The model under review builds one solid part; all positions refer to its coordinate system, in mm. Face numbers are marked on the shaded views. A direction names the side the tool comes from. Round coordinates to 2 decimals unless told otherwise and drop trailing zeros. Write each loop counter-clockwise with the first axis right and the second up, starting at its lowest first coordinate (ties: lowest second). Pieces come first, ordered by that corner, then holes. Notation, with made-up numbers: (17.25, -39.5) -> (44.25, -39.5) arc R25 cw to (44.25, -3.5) -> close; hole circle Ø9 at (-16, 44.25). An arc over 180 degrees is marked (long way). Answer as a JSON object with one key per item and string values. Group by question number.
1) Mouldability with a two-part tool opening along X and no side actions: class the marked faces 6, 7, 8 and 9 as pulls with the +X half, pulls with the -X half, needs draft (parallel to the pull), parting line crosses it, or undercut.
2) We need section C-C, the plane z = 15. Count the separate pieces of the cut face and the enclosed holes in it, then the cut area to 3 significant figures.
3) Machinability: for the marked faces 1, 2, 3, 4 and 5, which of the approach directions +Z, -Z, +X, -X, +Y, -Y give a long, thin tool a straight path to every point of the face, cutting with its end or side? Answer none if there is none.
4) We need section D-D, the plane x = 23. Write out the cut boundary in (y, z), then the cut area to 3 significant figures.
5) We need section A-A, the plane x = 18. Write out the cut boundary in (y, z).
6) We need section B-B, the plane y = 11.25. Write out the cut boundary in (x, z).
7) Insertion check: pin 1 Ø4 at (x, y) = (14.5, 6.5) entering from +Z; pin 2 Ø6 at (x, z) = (23, 21) entering from -Y; pin 3 Ø5 at (x, y) = (18.5, 6.5) entering from +Z. Each pin has a flat end and moves straight along its axis. Give the tip position at first contact, or say it passes through.
8) To check wall thickness, follow probe 1 along Y at (x, z) = (18, 4.65); probe 2 along Y at (x, z) = (18, 1.6); probe 3 along X at (y, z) = (21.25, 18.5). State the ranges of each line that lie inside material, in increasing order. Write a range as [from, to].
from build123d import *

# Parameters (mm, degrees)
SKETCH1_W                                           = 36
SKETCH1_H                                           = 24
BOSS_EXTRUDE1_DEPTH                                 = 6
CBORE_FOR_M3_HEX_SOCKET_HEAD_CAP_SCREW1_D           = 3.6
CBORE_FOR_M3_HEX_SOCKET_HEAD_CAP_SCREW1_DEPTH       = 12
CBORE_FOR_M3_HEX_SOCKET_HEAD_CAP_SCREW1_CBORE_D     = 6.5
CBORE_FOR_M3_HEX_SOCKET_HEAD_CAP_SCREW1_CBORE_DEPTH = 3.4
CBORE_FOR_M3_HEX_SOCKET_HEAD_CAP_SCREW1_TIP         = 1.081549114
BOSS_EXTRUDE2_DEPTH                                 = 19.5
SKETCH5_W                                           = 4.85
SKETCH5_H                                           = 8
CUT_EXTRUDE1_DEPTH                                  = 48.457876059
F_4_3_4_3_DIAMETER_HOLE1_D                          = 4.3
F_4_3_4_3_DIAMETER_HOLE1_DEPTH                      = 16
F_4_3_4_3_DIAMETER_HOLE1_TIP                        = 1.291850331
FILLET1_R                                           = 1
CHAMFER1_SIZE                                       = 2
CHAMFER2_SIZE                                       = 1


with BuildPart() as part:
    # Sketch1 → Boss-Extrude1 (new body)
    with BuildSketch(Plane.XY):
        with Locations((18, 12)):
            Rectangle(SKETCH1_W, SKETCH1_H)
    extrude(amount=BOSS_EXTRUDE1_DEPTH)

    # CBORE for M3 Hex Socket Head Cap Screw1
    with Locations(Plane.XY.offset(6)):
        with Locations((18, 17), (18, 7)):
            CounterBoreHole(CBORE_FOR_M3_HEX_SOCKET_HEAD_CAP_SCREW1_D / 2, CBORE_FOR_M3_HEX_SOCKET_HEAD_CAP_SCREW1_CBORE_D / 2, CBORE_FOR_M3_HEX_SOCKET_HEAD_CAP_SCREW1_CBORE_DEPTH, depth=CBORE_FOR_M3_HEX_SOCKET_HEAD_CAP_SCREW1_DEPTH)
            with Locations((0, 0, -(CBORE_FOR_M3_HEX_SOCKET_HEAD_CAP_SCREW1_DEPTH + CBORE_FOR_M3_HEX_SOCKET_HEAD_CAP_SCREW1_TIP / 2))):  # 118° drill point
                Cone(0, CBORE_FOR_M3_HEX_SOCKET_HEAD_CAP_SCREW1_D / 2, CBORE_FOR_M3_HEX_SOCKET_HEAD_CAP_SCREW1_TIP, mode=Mode.SUBTRACT)

    # Sketch4 → Boss-Extrude2 (add)
    with BuildSketch(Plane.XY.offset(6)):
        Polygon((7.85, 24), (0, 24), (0, 16), (4.85, 16), (4.85, 8), (0, 8), (0, 0), (7.85, 0), align=None)
        Polygon((36, 24), (28.15, 24), (28.15, 0), (36, 0), (36, 8), (31.15, 8), (31.15, 16), (36, 16), align=None)
    extrude(amount=BOSS_EXTRUDE2_DEPTH)

    # Sketch5 → Cut-Extrude1 (cut, through all)
    with BuildSketch(Plane.XY.offset(6)):
        with Locations((33.575, 12)):
            Rectangle(SKETCH5_W, SKETCH5_H)
        with Locations((2.425, 12)):
            Rectangle(SKETCH5_W, SKETCH5_H)
    extrude(amount=-CUT_EXTRUDE1_DEPTH, mode=Mode.SUBTRACT)

    # Ø4.3 (4.3) Diameter Hole1
    with Locations(Plane.XY.offset(25.5)):
        with Locations((3.925, 20), (3.925, 4), (32.075, 4), (32.075, 20)):
            Hole(F_4_3_4_3_DIAMETER_HOLE1_D / 2, depth=F_4_3_4_3_DIAMETER_HOLE1_DEPTH)
            with Locations((0, 0, -(F_4_3_4_3_DIAMETER_HOLE1_DEPTH + F_4_3_4_3_DIAMETER_HOLE1_TIP / 2))):  # 118° drill point
                Cone(0, F_4_3_4_3_DIAMETER_HOLE1_D / 2, F_4_3_4_3_DIAMETER_HOLE1_TIP, mode=Mode.SUBTRACT)

    # Fillet1
    fillet1_edges = [part.edges().sort_by_distance(p)[0] for p in [
        (0, 16, 12.75),
        (4.85, 16, 12.75),
        (4.85, 8, 12.75),
        (0, 8, 12.75),
        (36, 8, 12.75),
        (31.15, 8, 12.75),
        (31.15, 16, 12.75),
        (36, 16, 12.75),
        (0, 24, 12.75),
        (36, 24, 12.75),
        (36, 0, 12.75),
        (0, 0, 12.75),
    ]]
    fillet(fillet1_edges, radius=FILLET1_R)

    # Chamfer1
    chamfer1_edges = [part.edges().sort_by_distance(p)[0] for p in [
        (7.85, 0, 15.75),
        (7.85, 24, 15.75),
        (28.15, 24, 15.75),
        (28.15, 0, 15.75),
    ]]
    chamfer(chamfer1_edges, length=CHAMFER1_SIZE)

    # Chamfer2
    chamfer2_edges = [part.edges().sort_by_distance(p)[0] for p in [
        (28.15, 12, 25.5),
        (7.85, 12, 25.5),
    ]]
    chamfer(chamfer2_edges, length=CHAMFER2_SIZE)


solid = part.part
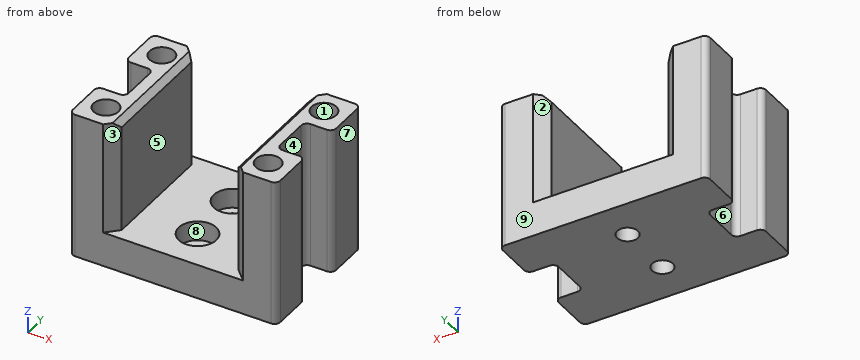
Here are the results:
{
 "1": {"face 6": "pulls with the -X half", "face 7": "pulls with the +X half", "face 8": "undercut", "face 9": "needs draft"},
 "2": {"separate pieces": "2", "enclosed holes": "4", "area": "232 mm^2"},
 "3": {"face 1": "+Z", "face 2": "+Z, +Y", "face 3": "+Z, -Y", "face 4": "+Z, -Z, +X", "face 5": "+Z, +Y, -Y"},
 "4": {"outline": "(0, 0) -> (24, 0) -> (24, 6) -> (0, 6) -> close", "area": "144 mm^2"},
 "5": {"outline": "(0, 0) -> (5.2, 0) -> (5.2, 2.6) -> (3.75, 2.6) -> (3.75, 6) -> (0, 6) -> close; (8.8, 0) -> (15.2, 0) -> (15.2, 2.6) -> (13.75, 2.6) -> (13.75, 6) -> (10.25, 6) -> (10.25, 2.6) -> (8.8, 2.6) -> close; (18.8, 0) -> (24, 0) -> (24, 6) -> (20.25, 6) -> (20.25, 2.6) -> (18.8, 2.6) -> close"},
 "6": {"outline": "(4.85, 0) -> (31.15, 0) -> (31.15, 25.5) -> (29.15, 25.5) -> (28.15, 24.5) -> (28.15, 6) -> (7.85, 6) -> (7.85, 24.5) -> (6.85, 25.5) -> (4.85, 25.5) -> close"},
 "7": {"pin 1": "stops at z = 6", "pin 2": "passes through", "pin 3": "stops at z = 2.6"},
 "8": {"probe 1": "y = [0, 3.75], [10.25, 13.75], [20.25, 24]", "probe 2": "y = [0, 5.2], [8.8, 15.2], [18.8, 24]", "probe 3": "x = [0, 2.18], [5.67, 7.85], [28.15, 30.33], [33.82, 36]"}
}
